```python
from build123d import *

# Parameters (mm, degrees)
SKETCH3_W               = 137.89
SKETCH3_H               = 284.48
BOSS_EXTRUDE1_DEPTH     = 109.22
BOSS_EXTRUDE1_DRAFT     = -2
FILLET1_R               = 17.272
CUT_EXTRUDE1_START      = 109.22
CUT_EXTRUDE1_DEPTH      = 40
CUT_EXTRUDE2_START      = 109.22
CUT_EXTRUDE2_DEPTH      = 13
CUT_EXTRUDE3_START      = 109.22
CUT_EXTRUDE3_DEPTH      = 18
CUT_EXTRUDE5_START      = 109.22
SKETCH1_6_R             = 8.35
CUT_EXTRUDE5_DEPTH      = 23
CUT_EXTRUDE7_START      = 109.22
SKETCH1_7_R             = 8.35
CUT_EXTRUDE7_DEPTH      = 31
FILLET2_R               = 2
CUT_EXTRUDE8_DEPTH      = 197.353435728
CUT_EXTRUDE8_DEPTH_BACK = 197.353435728


with BuildPart() as part:
    # Sketch3 → Boss-Extrude1 (with draft: the straight prism first)
    with BuildSketch(Plane(origin=(0, 0, 0), x_dir=(1, 0, 0), z_dir=(0, 1, 0))):
        Rectangle(SKETCH3_W, SKETCH3_H)
    extrude(amount=BOSS_EXTRUDE1_DEPTH)
    # Boss-Extrude1: the draft: its side faces are tilted about the plane it starts from
    boss_extrude1_sides = [part.faces().sort_by_distance(p)[0] for p in [
        (0, 54.61, 142.24),
        (68.945, 54.61, 0),
        (0, 54.61, -142.24),
        (-68.945, 54.61, 0),
    ]]
    draft(boss_extrude1_sides, Plane(origin=(0, 0, 0), x_dir=(1, 0, 0), z_dir=(0, 1, 0)), BOSS_EXTRUDE1_DRAFT)

    # Fillet1
    fillet1_edges = [part.edges().sort_by_distance(p)[0] for p in [
        (0, 0, 142.24),
        (0, 0, -142.24),
        (68.945, 0, 0),
        (70.852023222, 54.61, 144.147023222),
        (70.852023222, 54.61, -144.147023222),
    ]]
    fillet(fillet1_edges, radius=FILLET1_R)

    # Sketch1 → Cut-Extrude1 (cut)
    with BuildSketch(Plane(origin=(0, 0, 0), x_dir=(1, 0, 0), z_dir=(0, 1, 0)).offset(CUT_EXTRUDE1_START)):
        with BuildLine():
            Line((43.981048837, 90.304046444), (56.381048837, 90.304046444))
            Line((56.381048837, 90.304046444), (56.381048837, 77.504046444))
            Line((56.381048837, 77.504046444), (43.981048837, 77.504046444))
            ThreePointArc((43.981048837, 77.504046444), (-54.503046444, 83.904046444), (43.981048837, 90.304046444))
        make_face()
        with BuildLine():
            Line((43.981048837, -77.504046444), (56.381048837, -77.504046444))
            Line((56.381048837, -77.504046444), (56.381048837, -90.304046444))
            Line((56.381048837, -90.304046444), (43.981048837, -90.304046444))
            ThreePointArc((43.981048837, -90.304046444), (-54.503046444, -83.904046444), (43.981048837, -77.504046444))
        make_face()
    extrude(amount=-CUT_EXTRUDE1_DEPTH, mode=Mode.SUBTRACT)

    # Sketch1<4> → Cut-Extrude2 (cut)
    with BuildSketch(Plane(origin=(0, 0, 0), x_dir=(1, 0, 0), z_dir=(0, 1, 0)).offset(CUT_EXTRUDE2_START)):
        with BuildLine():
            Line((-25.038870367, -15.216738709), (-32.81704496, -7.438564116))
            ThreePointArc((-32.81704496, -7.438564116), (-55.423049532, 10.217692988), (-37.766792428, -12.388311584))
            Line((-37.766792428, -12.388311584), (-29.988617835, -20.166486177))
            Line((-29.988617835, -20.166486177), (-25.038870367, -15.216738709))
        make_face()
    extrude(amount=-CUT_EXTRUDE2_DEPTH, mode=Mode.SUBTRACT)

    # Sketch1<5> → Cut-Extrude3 (cut)
    with BuildSketch(Plane(origin=(0, 0, 0), x_dir=(1, 0, 0), z_dir=(0, 1, 0)).offset(CUT_EXTRUDE3_START)):
        with BuildLine():
            Line((-23.058973173, 19.589272149), (-15.492930614, 12.02322959))
            ThreePointArc((-15.492930614, 12.02322959), (16.187867493, -14.707821049), (-10.543183146, 16.972977058))
            Line((-10.543183146, 16.972977058), (-18.109225705, 24.539019617))
            Line((-18.109225705, 24.539019617), (-23.058973173, 19.589272149))
        make_face()
    extrude(amount=-CUT_EXTRUDE3_DEPTH, mode=Mode.SUBTRACT)

    # Sketch1<6> → Cut-Extrude5 (cut)
    # profile 1 of 2: a face of its own
    with BuildSketch(Plane(origin=(0, 0, 0), x_dir=(1, 0, 0), z_dir=(0, 1, 0)).offset(CUT_EXTRUDE5_START)):
        with BuildLine():
            Line((38.583046444, 12.7), (56.583046444, 12.7))
            ThreePointArc((56.583046444, 12.7), (60.11858035, 14.164466094), (61.583046444, 17.7))
            Line((61.583046444, 17.7), (61.583046444, 35.7))
            ThreePointArc((61.583046444, 35.7), (60.11858035, 39.235533906), (56.583046444, 40.7))
            Line((56.583046444, 40.7), (38.583046444, 40.7))
            ThreePointArc((38.583046444, 40.7), (35.047512538, 39.235533906), (33.583046444, 35.7))
            Line((33.583046444, 35.7), (33.583046444, 17.7))
            ThreePointArc((33.583046444, 17.7), (35.047512538, 14.164466094), (38.583046444, 12.7))
        make_face()
        with Locations(Location((47.583046444, 26.7, 0), (0, 0, 90))):
            Circle(SKETCH1_6_R, mode=Mode.SUBTRACT)
    # profile 2 of 2: a face of its own
    with BuildSketch(Plane(origin=(0, 0, 0), x_dir=(1, 0, 0), z_dir=(0, 1, 0)).offset(CUT_EXTRUDE5_START)):
        with BuildLine():
            Line((38.583046444, -40.7), (56.583046444, -40.7))
            ThreePointArc((56.583046444, -40.7), (60.11858035, -39.235533906), (61.583046444, -35.7))
            Line((61.583046444, -35.7), (61.583046444, -17.7))
            ThreePointArc((61.583046444, -17.7), (60.11858035, -14.164466094), (56.583046444, -12.7))
            Line((56.583046444, -12.7), (38.583046444, -12.7))
            ThreePointArc((38.583046444, -12.7), (35.047512538, -14.164466094), (33.583046444, -17.7))
            Line((33.583046444, -17.7), (33.583046444, -35.7))
            ThreePointArc((33.583046444, -35.7), (35.047512538, -39.235533906), (38.583046444, -40.7))
        make_face()
        with Locations(Location((47.583046444, -26.7, 0), (0, 0, 90))):
            Circle(SKETCH1_6_R, mode=Mode.SUBTRACT)
    extrude(amount=-CUT_EXTRUDE5_DEPTH, mode=Mode.SUBTRACT)

    # Sketch1<7> → Cut-Extrude7 (cut)
    with BuildSketch(Plane(origin=(0, 0, 0), x_dir=(1, 0, 0), z_dir=(0, 1, 0)).offset(CUT_EXTRUDE7_START)):
        with Locations(Location((47.583046444, 26.7, 0), (0, 0, 90))):
            Circle(SKETCH1_7_R)
        with Locations(Location((47.583046444, -26.7, 0), (0, 0, 90))):
            Circle(SKETCH1_7_R)
    extrude(amount=-CUT_EXTRUDE7_DEPTH, mode=Mode.SUBTRACT)

    # Fillet2
    fillet2_edges = [part.edges().sort_by_distance(p)[0] for p in [
        (43.981048837, 89.22, -77.504046444),
        (43.981048837, 89.22, -90.304046444),
        (56.381048837, 89.22, -90.304046444),
        (56.381048837, 89.22, -77.504046444),
        (43.981048837, 89.22, 90.304046444),
        (43.981048837, 89.22, 77.504046444),
        (56.381048837, 89.22, 77.504046444),
        (56.381048837, 89.22, 90.304046444),
        (-25.038870367, 102.72, 15.216738709),
        (-29.988617835, 102.72, 20.166486177),
        (-37.766792428, 102.72, 12.388311584),
        (-32.81704496, 102.72, 7.438564116),
        (-23.058973173, 100.22, -19.589272149),
        (-18.109225705, 100.22, -24.539019617),
        (-10.543183146, 100.22, -16.972977058),
        (-15.492930614, 100.22, -12.02322959),
    ]]
    fillet(fillet2_edges, radius=FILLET2_R)

    # Sketch4 → Cut-Extrude8 (cut, two sides: drawn at the far end of the back side and taken through both)
    with BuildSketch(Plane.XY.offset(-CUT_EXTRUDE8_DEPTH_BACK)):
        Polygon((-68.945, 109.22), (-68.945, 0), (-84.208745504, 109.22), align=None)
    extrude(amount=CUT_EXTRUDE8_DEPTH + CUT_EXTRUDE8_DEPTH_BACK, mode=Mode.SUBTRACT)


solid = part.part
```
Check sheet for the modelled part. Datum: model origin and axes. Units: mm. Round coordinates to 2 decimals unless told otherwise and drop trailing zeros. Loops run counter-clockwise (first coordinate to the right, second up) from the corner with the lowest first, then second, coordinate; pieces in that order, holes last. Notation, with made-up numbers: (-9.75, 18.5) - (29.25, 18.5) arc R23 ccw to (29.25, 35.5) - close; hole circle Ø1 at (82, -16.75). An arc over 180 degrees is marked (long way). Write item = value, one per line. Start each with the question number.
Q1. Section check A-A (z = -26.7). Record the boundary of the cut face in (x, y) (3 decimals), plus the area to 3 significant figures.
Q2. Depth check by flat-ended pin: P1, Ø2.5, axis at x = 51, y = 94.5, coming from the -Z side; P2, Ø5.5, axis at y = 93, z = 22.5, coming from the +X side; P3, Ø20, axis at y = 94, z = -29, coming from the +X side. Enter the tip coordinate at first touch or a pass-through.
Q3. Section check D-D (z = 115.5). Record the boundary of the cut face in (x, y) (3 decimals).
Q4. Release check for a two-part mould opening along Z. For faces 1 (the face through (-68.945, 55, -2)), 2 (the face through (-7.491, 4.977, -137.692)), 3 (the face through (-54.46, 89.5, 85.96)), 4 (the face through (0, 91.22, -2)) record: pulls with the +Z half, pulls with the -Z half, needs draft (parallel to the pull), parting line crosses it, or undercut.
Q5. Section check C-C (z = 62). Record the boundary of the cut face in (x, y) (3 decimals), plus the area to 3 significant figures.
Q6. Thickness scan on L1, parallel to Z at x = 47, y = 70.5; L2, parallel to Z at x = 21, y = 73; L3, parallel to Z at x = -14, y = 101. Record the ranges inside material, lowest first.
Q7. Section check B-B (x = 14.5). Record the boundary of the cut face in (y, z), plus the area to 3 significant figures.
Derived:
q1.outline = (-68.945, 0) - (52.266, 0) arc R17.272 ccw to (69.527, 16.669) - (72.759, 109.22) - (61.583, 109.22) - (61.583, 86.22) - (55.933, 86.22) - (55.933, 78.22) - (39.233, 78.22) - (39.233, 86.22) - (33.583, 86.22) - (33.583, 109.22) - (-68.945, 109.22) - close
q1.area = 14,400 mm^2
q2.P1 = -145.58
q2.P2 = 72.29
q2.P3 = 72.58
q3.outline = (-68.945, 0) - (52.266, 0) arc R17.272 ccw to (69.527, 16.669) - (72.759, 109.22) - (32.986, 109.22) - (32.986, 69.22) - (-43.092, 69.22) - (-43.092, 109.22) - (-68.945, 109.22) - close
q4.face_1 = needs draft
q4.face_2 = pulls with the -Z half
q4.face_3 = undercut
q4.face_4 = undercut
q5.outline = (-68.945, 0) - (52.266, 0) arc R17.272 ccw to (69.527, 16.669) - (72.759, 109.22) - (39.281, 109.22) - (39.281, 69.22) - (-49.387, 69.22) - (-49.387, 109.22) - (-68.945, 109.22) - close
q5.area = 11,700 mm^2
q6.L1 = -144.7 to -90.3, -77.5 to 77.5, 90.3 to 144.7
q6.L2 = -144.79 to -125.93, -41.87 to 41.87, 125.93 to 144.79
q6.L3 = -145.77 to -132.54, -35.27 to -20.43, 13.89 to 35.27, 132.54 to 145.77
q7.outline = (0, -125.56) arc R17.27 ccw to (16.67, -142.82) - (109.22, -146.05) - (109.22, -129.32) - (69.22, -129.32) - (69.22, -38.48) - (109.22, -38.48) - (109.22, -16.22) - (91.22, -16.22) - (91.22, 16.22) - (109.22, 16.22) - (109.22, 38.48) - (69.22, 38.48) - (69.22, 129.32) - (109.22, 129.32) - (109.22, 146.05) - (16.67, 142.82) arc R17.27 ccw to (0, 125.56) - close
q7.area = 23,500 mm^2
